```python
from build123d import *

# Parameters (mm, degrees)
SKETCH1_W           = 150
SKETCH1_H           = 150
BOSS_EXTRUDE1_DEPTH = 2
CUT_EXTRUDE2_REACH  = 4
SKETCH4_W           = 20
SKETCH4_H           = 15
CUT_EXTRUDE3_REACH  = 4
SKETCH7_W           = 66
SKETCH7_H           = 19


with BuildPart() as part:
    # Sketch1 → Boss-Extrude1 (new body)
    with BuildSketch(Plane(origin=(0, 0, 0), x_dir=(1, 0, 0), z_dir=(0, 1, 0))):
        Rectangle(SKETCH1_W, SKETCH1_H)
    extrude(amount=BOSS_EXTRUDE1_DEPTH)

    # Sketch4 → Cut-Extrude2 (cut, up to next)
    with BuildSketch(Plane(origin=(0, 2, 0), x_dir=(1, 0, 0), z_dir=(0, 1, 0)), mode=Mode.PRIVATE) as cut_extrude2_sk1:
        with Locations((-65, 0.5)):
            Rectangle(SKETCH4_W, SKETCH4_H)
    cut_extrude2_tool1 = extrude(cut_extrude2_sk1.sketch, amount=-CUT_EXTRUDE2_REACH, mode=Mode.PRIVATE) & part.part
    add(cut_extrude2_tool1.solids().sort_by_distance((-65, 2, -0.5))[0], mode=Mode.SUBTRACT)

    # Sketch7 → Cut-Extrude3 (cut, up to next)
    with BuildSketch(Plane.XZ, mode=Mode.PRIVATE) as cut_extrude3_sk1:
        with Locations((42, 65.5)):
            Rectangle(SKETCH7_W, SKETCH7_H)
    cut_extrude3_tool1 = extrude(cut_extrude3_sk1.sketch, amount=-CUT_EXTRUDE3_REACH, mode=Mode.PRIVATE) & part.part
    add(cut_extrude3_tool1.solids().sort_by_distance((42, 0, 65.5))[0], mode=Mode.SUBTRACT)
    # Sketch7 → Cut-Extrude3 (cut, up to next)
    with BuildSketch(Plane.XZ, mode=Mode.PRIVATE) as cut_extrude3_sk2:
        with Locations((42, -65.5)):
            Rectangle(SKETCH7_W, SKETCH7_H)
    cut_extrude3_tool2 = extrude(cut_extrude3_sk2.sketch, amount=-CUT_EXTRUDE3_REACH, mode=Mode.PRIVATE) & part.part
    add(cut_extrude3_tool2.solids().sort_by_distance((42, 0, -65.5))[0], mode=Mode.SUBTRACT)


solid = part.part
```
For this review, take the finished solid that the model builds, in its own axes (mm). Round coordinates to 2 decimals unless told otherwise and drop trailing zeros. Write each loop counter-clockwise with the first axis right and the second up, starting at its lowest first coordinate (ties: lowest second). Pieces come first, ordered by that corner, then holes. Notation, with made-up numbers: (33, 38) - (60, 38) arc R21 cw to (60, 53) - close; hole circle Ø8 at (-5, -33). An arc over 180 degrees is marked (long way). Put each result on its own line as item: value.
Q1. Insertion check: pin 1 Ø1 at (y, z) = (1, -66) entering from +X; pin 2 Ø0.6 at (x, y) = (29.5, 0.5) entering from +Z. Each pin has a flat end and moves straight along its axis. Give the tip position at first contact, or say it passes through.
Solved:
pin 1: stops at x = 9
pin 2: stops at z = 56
Q2. We need section B-B (z = 59.5). Give the boundary of the cut face in (x, y), and give its area (3 significant figures).
Solved:
outline: (-75, 0) - (9, 0) - (9, 2) - (-75, 2) - close
area: 168 mm2
Q3. Wall thickness on probe 1 along Z at (x, y) = (-64.5, 0.65); probe 2 along Z at (x, y) = (23, 1.85); probe 3 along X at (y, z) = (0.65, 60): over which ranges is each line inside the solid? List them lowest first.
Solved:
probe 1: z = -75 to -8, 7 to 75
probe 2: z = -56 to 56
probe 3: x = -75 to 9
Q4. We need section A-A (y = 1.65). Give the boundary of the cut face in (x, z).
Solved:
outline: (-75, -75) - (9, -75) - (9, -56) - (75, -56) - (75, 56) - (9, 56) - (9, 75) - (-75, 75) - (-75, 7) - (-55, 7) - (-55, -8) - (-75, -8) - close
Q5. We need section C-C (x = 31). Give the boundary of the cut face in (y, z), and give its area (3 significant figures).
Solved:
outline: (0, -56) - (2, -56) - (2, 56) - (0, 56) - close
area: 224 mm2
